```python
from build123d import *

# Parameters (mm, degrees)
F0_W           = 10
F0_H           = 53
F0_W_2         = 310
F1_DEPTH       = 10
F3_D           = 3.5
F3_CBORE_D     = 7
F3_CBORE_DEPTH = 5
F4_R           = 1.25
F5_DEPTH       = 53


with BuildPart() as f1:
    # F0 (on Top) → F1 (new body)
    with BuildSketch(Plane.XY):
        with Locations((-224.1861552, -33.3002303571)):
            Rectangle(F0_W, F0_H)
        Polygon((-39.1861552, -6.8002303571), (-219.1861552, -6.8002303571), (-219.1861552, -59.8002303571), (-218.1861552, -59.8002303571), (-218.1861552, -47.8002303571), (-40.1861552, -47.8002303571), (-40.1861552, -59.8002303571), (-39.1861552, -59.8002303571), align=None)
        with Locations((-34.1861552, -33.3002303571)):
            Rectangle(F0_W, F0_H)
        with Locations((125.8138448, -33.3002303571)):
            Rectangle(F0_W_2, F0_H)
    extrude(amount=F1_DEPTH)

    # F3 (through all)
    with Locations(Plane.XY.offset(10)):
        with Locations((-224.1861552, -21.8002303571), (-224.1861552, -44.8002303571), (-34.1861620545, -21.8002303571), (-34.1861620545, -44.8002303571)):
            CounterBoreHole(F3_D / 2, F3_CBORE_D / 2, F3_CBORE_DEPTH)

    # F4 (on face) → F5 (cut, through all)
    with BuildSketch(Plane(origin=(0, -6.8002303571, 0), x_dir=(-1, 0, 0), z_dir=(0, 1, 0))):
        with Locations((-180.8138448, 5)):
            Circle(F4_R)
        with Locations((-70.8138448, 5)):
            Circle(F4_R)
        with Locations((79.1861552, 5)):
            Circle(F4_R)
        with Locations((129.1861552, 5)):
            Circle(F4_R)
        with Locations((179.1861552, 5)):
            Circle(F4_R)
    extrude(amount=-F5_DEPTH, mode=Mode.SUBTRACT)


solid = f1.part
```
Model file for the job. Use its own axes, mm. A direction names the side the tool comes from. Coordinates: 2 decimals unless noted, no trailing zeros. Write each loop counter-clockwise with the first axis right and the second up, starting at its lowest first coordinate (ties: lowest second). Pieces come first, ordered by that corner, then holes. Notation, with made-up numbers: (4.25, -39.5) - (28.25, -39.5) arc R18 cw to (28.25, -22.5) - close; hole circle Ø10 at (46.5, -5.75). An arc over 180 degrees is marked (long way). One line per item, written item: value. Start each with the question number.
1. Slice it at A-A (y = -53). Write the cut outline in (x, z), plus the area to 3 significant figures.
2. Mould opens along X. For faces 1 (the flat face through (-130.4, -47.8, 6)), 2 (the flat face through (-229.186, -34, 5)), 3 (the flat face through (29, -6.8, 5)) say: released by +X, released by -X, zero draft, split by the parting line, or undercut.
3. Probe line 1 (X direction, y = -33, z = 4.5); line 2 (X direction, y = -34, z = 6); line 3 (X direction, y = -50, z = 9.75). List the from-to ranges inside material, lowest first. Write a range as from..to.
4. Tool access for faces 4 (the flat face through (-218.186, -54, 5)), 5 (the flat face through (280.814, -34, 5)): list every direction of +Z, -Z, +X, -X, +Y, -Y with a clear straight run to the whole face (end or side of a thin tool).
5. Flat gauge pins, fed straight in: pin 1 (5 mm diameter, centred on x = -154.5, z = 2.5, fed in from -Y); pin 2 (3.5 mm diameter, centred on x = -224, y = -22.5, fed in from +Z). Where does each tip first touch, or does it go through?
Answers below:
1. outline: (-229.19, 0) - (-218.19, 0) - (-218.19, 10) - (-229.19, 10) - close; (-40.19, 0) - (280.81, 0) - (280.81, 10) - (-40.19, 10) - close; hole circle Ø2.5 at (70.81, 5); hole circle Ø2.5 at (180.81, 5)
1. area: 3,310 mm^2
2. face 1: undercut
2. face 2: released by -X
2. face 3: zero draft
3. line 1: x = -229.19..-180.33, -178.04..-130.33, -128.04..-80.33, -78.04..69.67, 71.96..179.67, 181.96..280.81
3. line 2: x = -229.19..-179.94, -178.44..-129.94, -128.44..-79.94, -78.44..70.06, 71.56..180.06, 181.56..280.81
3. line 3: x = -229.19..-218.19, -40.19..280.81
4. face 4: +Z, -Z, -Y
4. face 5: +Z, -Z, +X, +Y, -Y
5. pin 1: stops at y = -47.8
5. pin 2: stops at z = 5
